```python
from build123d import *

# Parameters (mm, degrees)
SKETCH_1_W          = 90
SKETCH_1_H          = 90
EXTRUDE_1_DEPTH     = 6
SKETCH_2_R          = 1.35
CUT_EXTRUDE_1_DEPTH = 6
SKETCH_3_R          = 2.6
CUT_EXTRUDE_2_DEPTH = 6
SKETCH_4_R          = 1.6
CUT_EXTRUDE_3_DEPTH = 6
FILLET_1_R          = 10


with BuildPart() as part:
    # 草图1 → 凸台-拉伸1 (new body)
    with BuildSketch(Plane(origin=(0, 0, 0), x_dir=(1, 0, 0), z_dir=(0, 1, 0))):
        Rectangle(SKETCH_1_W, SKETCH_1_H)
    extrude(amount=EXTRUDE_1_DEPTH)

    # 草图2 → 切除-拉伸1 (cut)
    with BuildSketch(Plane(origin=(0, 6, 0), x_dir=(1, 0, 0), z_dir=(0, 1, 0))):
        with Locations(Location((-29, 7.5, 0), (0, 0, 270))):
            Circle(SKETCH_2_R)
        with Locations(Location((-29, -41.5, 0), (0, 0, 270))):
            Circle(SKETCH_2_R)
        with Locations(Location((-18, 1, 0), (0, 0, 270))):
            Circle(SKETCH_2_R)
        with Locations(Location((-18, -35, 0), (0, 0, 270))):
            Circle(SKETCH_2_R)
        with Locations(Location((18, -35, 0), (0, 0, 270))):
            Circle(SKETCH_2_R)
        with Locations(Location((29, -41.5, 0), (0, 0, 270))):
            Circle(SKETCH_2_R)
        with Locations(Location((18, 1, 0), (0, 0, 270))):
            Circle(SKETCH_2_R)
        with Locations(Location((29, 7.5, 0), (0, 0, 270))):
            Circle(SKETCH_2_R)
    extrude(amount=-CUT_EXTRUDE_1_DEPTH, mode=Mode.SUBTRACT)

    # 草图3 → 切除-拉伸2 (cut)
    with BuildSketch(Plane(origin=(0, 6, 0), x_dir=(1, 0, 0), z_dir=(0, 1, 0))):
        with Locations(Location((0, 25.05, 0), (0, 0, 270))):
            Circle(SKETCH_3_R)
    extrude(amount=-CUT_EXTRUDE_2_DEPTH, mode=Mode.SUBTRACT)

    # 草图4 → 切除-拉伸3 (cut)
    with BuildSketch(Plane(origin=(0, 6, 0), x_dir=(1, 0, 0), z_dir=(0, 1, 0))):
        with Locations(Location((-40, -35, 0), (0, 0, 270))):
            Circle(SKETCH_4_R)
        with Locations(Location((-40, 35, 0), (0, 0, 90))):
            Circle(SKETCH_4_R)
    extrude(amount=-CUT_EXTRUDE_3_DEPTH, mode=Mode.SUBTRACT)

    # 圆角1
    fillet_1_edges = [part.edges().sort_by_distance(p)[0] for p in [
        (45, 3, 45),
        (45, 3, -45),
    ]]
    fillet(fillet_1_edges, radius=FILLET_1_R)


solid = part.part
```
Input: part model. Units: mm. Frame: model coordinates. Round coordinates to 2 decimals unless told otherwise and drop trailing zeros. Loops run counter-clockwise (first coordinate to the right, second up) from the corner with the lowest first, then second, coordinate; pieces in that order, holes last.
1) Section query A-A on x = -29. Return the cut outline in (y, z), plus the area to 3 significant figures.
Ans:
outline: (0, -45) - (6, -45) - (6, -8.85) - (0, -8.85) - close; (0, -6.15) - (6, -6.15) - (6, 40.15) - (0, 40.15) - close; (0, 42.85) - (6, 42.85) - (6, 45) - (0, 45) - close
area: 508 mm2
2) Section query B-B on z = -25.05. Return the cut outline in (x, y).
Ans:
outline: (-45, 0) - (-2.6, 0) - (-2.6, 6) - (-45, 6) - close; (2.6, 0) - (45, 0) - (45, 6) - (2.6, 6) - close
3) Section query D-D on z = -7.5. Return the cut outline in (x, y).
Ans:
outline: (-45, 0) - (-30.35, 0) - (-30.35, 6) - (-45, 6) - close; (-27.65, 0) - (27.65, 0) - (27.65, 6) - (-27.65, 6) - close; (30.35, 0) - (45, 0) - (45, 6) - (30.35, 6) - close
4) Material intervals for line 1 (X direction, y = 4.8, z = 35); line 2 (X direction, y = 3.5, z = -7.5); line 3 (X direction, y = 3.3, z = -35), sorted ascending.
Ans:
line 1: x = -45 to -41.6, -38.4 to -19.35, -16.65 to 16.65, 19.35 to 45
line 2: x = -45 to -30.35, -27.65 to 27.65, 30.35 to 45
line 3: x = -45 to -41.6, -38.4 to 45
5) Pin query (flat end, axial travel): pin 1 (1.6 mm diameter, centred on x = 18, z = -1, fed in from -Y). Return the tip coordinate at first contact, or that it passes through.
Ans:
pin 1: passes through
6) Section query C-C on y = 2.3. Count the separate pieces of the cut face and the enclosed holes in it, plus the area to 3 significant figures.
Ans:
separate pieces: 1
enclosed holes: 11
area: 7,970 mm2
